```python
from build123d import *

# Parameters (mm, degrees)
SKETCH1_W           = 85
SKETCH1_H           = 45
BOSS_EXTRUDE1_DEPTH = 2.5
BOSS_EXTRUDE2_DEPTH = 50
BOSS_EXTRUDE3_DEPTH = 58.743328
SKETCH4_W           = 35
SKETCH4_H           = 45
SKETCH4_R           = 16.1
BOSS_EXTRUDE4_DEPTH = 7
HOLE1_D             = 4.2
HOLE1_DEPTH         = 20
HOLE1_CBORE_D       = 7
HOLE1_CBORE_DEPTH   = 5
FILLET4_R           = 3
FILLET5_R           = 3
FILLET6_R           = 3
FILLET7_R           = 0.58


with BuildPart() as part:
    # Sketch1 → Boss-Extrude1 (new body)
    with BuildSketch(Plane(origin=(0, 0, 0), x_dir=(1, 0, 0), z_dir=(0, 1, 0))):
        with Locations((-42.5, 22.5)):
            Rectangle(SKETCH1_W, SKETCH1_H)
    extrude(amount=BOSS_EXTRUDE1_DEPTH)

    # Sketch2 → Boss-Extrude2 (add)
    with BuildSketch(Plane(origin=(0, 0, 0), x_dir=(0, 0, -1), z_dir=(1, 0, 0))):
        Polygon((0, 2.5), (45, 40.259483403), (45, 2.5), align=None)
    extrude(amount=-BOSS_EXTRUDE2_DEPTH)

    # Sketch3 → Boss-Extrude3 (add)
    with BuildSketch(Plane(origin=(-50, 40.259483403, -45), x_dir=(1, 0, 0), z_dir=(0, -0.6427876096865354, 0.7660444431189815))):
        Polygon((0, 0), (0, 15), (8, 15), (6.5, 12), (5, 12), (5, 0), align=None)
    extrude(amount=BOSS_EXTRUDE3_DEPTH)

    # Sketch4 → Boss-Extrude4 (add)
    with BuildSketch(Plane(origin=(0, 2.5, 0), x_dir=(1, 0, 0), z_dir=(0, 1, 0))):
        with Locations((-67.5, 22.5)):
            Rectangle(SKETCH4_W, SKETCH4_H)
        with Locations(Location((-67.5, 22.5, 0), (0, 0, 270))):
            Circle(SKETCH4_R, mode=Mode.SUBTRACT)
    extrude(amount=BOSS_EXTRUDE4_DEPTH)

    # Hole1
    with Locations(Plane(origin=(-80, 9.5, -40), x_dir=(0, 0, 1), z_dir=(0, 1, 0))):
        with Locations((0, 0), (35, 0)):
            CounterBoreHole(HOLE1_D / 2, HOLE1_CBORE_D / 2, HOLE1_CBORE_DEPTH, depth=HOLE1_DEPTH)

    # Sketch8 → Cut-Revolve1 (revolve, cut)
    with BuildSketch(Plane.XY.offset(-22.5), mode=Mode.PRIVATE) as cut_revolve1_sk:
        Polygon((-2.5, 21.379741701), (-2.5, 6), (-3.9, 6), (-3.9, -6.519563006), (-6, -6.519563006), (-6, 21.379741701), (-6, 29.263564953), (-2.5, 29.263564953), align=None)
    revolve(cut_revolve1_sk.sketch.rotate(Axis((-6, -6.519563006, -22.5), (0, 1, 0)), 90), axis=Axis((-6, -6.519563006, -22.5), (0, 1, 0)), mode=Mode.SUBTRACT)

    # Fillet4
    fillet4_edges = [part.edges().sort_by_distance(p)[0] for p in [
        (-50, 32.870408355, -12.858185862),
    ]]
    fillet(fillet4_edges, radius=FILLET4_R)

    # Fillet5
    fillet5_edges = [part.edges().sort_by_distance(p)[0] for p in [
        (-44.5, 51.75015005, -35.358185855),
        (-49.121320344, 51.077042382, -35.922990251),
        (-50, 44.855750062, -41.143274342),
        (-50, 24.879741701, -45),
    ]]
    fillet(fillet5_edges, radius=FILLET5_R)

    # Fillet6
    fillet6_edges = [part.edges().sort_by_distance(p)[0] for p in [
        (-44.5, 13.99066666, 9.64181413),
        (-49.121320344, 13.317558992, 9.077009734),
        (-50, 7.096266672, 3.856725643),
    ]]
    fillet(fillet6_edges, radius=FILLET6_R)

    # Fillet7
    fillet7_edges = [part.edges().sort_by_distance(p)[0] for p in [
        (-45, 21.379741708, -22.500000008),
        (-45, 30.572275025, -14.786548691),
    ]]
    fillet(fillet7_edges, radius=FILLET7_R)


solid = part.part
```
Part model, mm, in its own coordinate system. A direction names the side the tool comes from. Give positions to 0.01 mm unless a question says otherwise; leave off trailing zeros. Order: outer loops, then holes, each group sorted by start corner. A loop starts at its lowest first (then second) coordinate and runs counter-clockwise, first axis right, second up. Notation, with made-up numbers: M 46.25,10 L 85.25,10 A21 cw 85.25,37 Z; hole C -36,54.5 d10. An arc over 180 degrees is marked long. Use a Markdown table: item, result. Add a question column.
(1) 3-axis set-ups, long thin cutter, end or side, ignore diameter. For faces 1 (the face through (-82.1, 7, -42.8)), 2 (the face through (-81.278, 2.219, -3.334)), 3 (the face through (-44.46, 13.92, 8.4)), 4 (the face through (-49.14, 24.66, -44.1)), 5 (the face through (-43.954, 30.837, -15.102)): which of +Z, -Z, +X, -X, +Y, -Y reach the whole face in a straight line?
(2) Saw through at B-B, the plane x = -63. Give the cut face in (y, z).
(3) Drop flat-ended pins along their axis: P1, Ø10, axis at y = 27, z = -13.5, coming from the -X side; P2, Ø6.5, axis at x = -80, z = -5, coming from the +Y side; P3, Ø8, axis at y = 35.5, z = -23, coming from the +X side. Give the stop position or say it passes through.
(4) Saw through at A-A, the plane x = -80. Give the cut face in (y, z).
(5) Mould opens along Z. For faces 6 (the face through (-50, 21, -24)), 7 (the face through (-44.535, 33.108, -13.141)), 8 (the face through (-42.74, 32, -14.12)) say: +Z half, -Z half, draft (parallel to the pull), parting line (faces both ways), or undercut.
(6) Probe line 1 along X through (y, z) = (4, -22.5); line 2 along X through (y, z) = (2.7, -5); line 3 along Y through (x, z) = (-54, -40.5). List the from-to ranges inside material, lowest first. Write a range as [from, to].
(7) Saw through at C-C, the plane x = -35. Give the cut face in (y, z), and give its area (3 significant figures).
Answer key:
| question | item | result |
|---|---|---|
| 1 | face 1 | +Y |
| 1 | face 2 | +Y, -Y |
| 1 | face 3 | +Z, +X, -X |
| 1 | face 4 | -Z, -X, +Y |
| 1 | face 5 | +X |
| 2 | outline | M 0,-45 L 9.5,-45 L 9.5,-37.96 L 2.5,-37.96 L 2.5,-7.04 L 9.5,-7.04 L 9.5,0 L 0,0 Z |
| 3 | P1 | x = -50 |
| 3 | P2 | y = 4.5 |
| 3 | P3 | x = -42.25 |
| 4 | outline | M 0,-45 L 9.5,-45 L 9.5,-43.5 L 4.5,-43.5 L 4.5,-42.1 L 0,-42.1 Z; M 0,-37.9 L 4.5,-37.9 L 4.5,-36.5 L 9.5,-36.5 L 9.5,-32.65 L 2.5,-32.65 L 2.5,-12.35 L 9.5,-12.35 L 9.5,-8.5 L 4.5,-8.5 L 4.5,-7.1 L 0,-7.1 Z; M 0,-2.9 L 4.5,-2.9 L 4.5,-1.5 L 9.5,-1.5 L 9.5,0 L 0,0 Z |
| 5 | face 6 | draft |
| 5 | face 7 | +Z half |
| 5 | face 8 | undercut |
| 6 | line 1 | [-85, -83.6], [-51.4, -8.1], [-3.9, 0] |
| 6 | line 2 | [-85, -82.1], [-77.9, 0] |
| 6 | line 3 | [0, 9.5] |
| 7 | outline | M 0,-45 L 40.26,-45 L 2.5,0 L 0,0 Z |
| 7 | area | 962 mm^2 |
